Answer from the drawing. Dimensions are ordinates in mm from the lowest x, y and z of the part. A direction names the side the tool comes from. Coordinates: 2 decimals unless noted, no trailing zeros. Order: outer loops, then holes, each group sorted by start corner. A loop starts at its lowest first (then second) coordinate and runs counter-clockwise, first axis right, second up. Notation, with made-up numbers: (-13.5, 70.5) -> (31.5, 70.5) arc R22 cw to (31.5, 100.5) -> close; hole circle Ø11 at (-36, 82). An arc over 180 degrees is marked (long way). Answer in a Markdown table with one row per item.
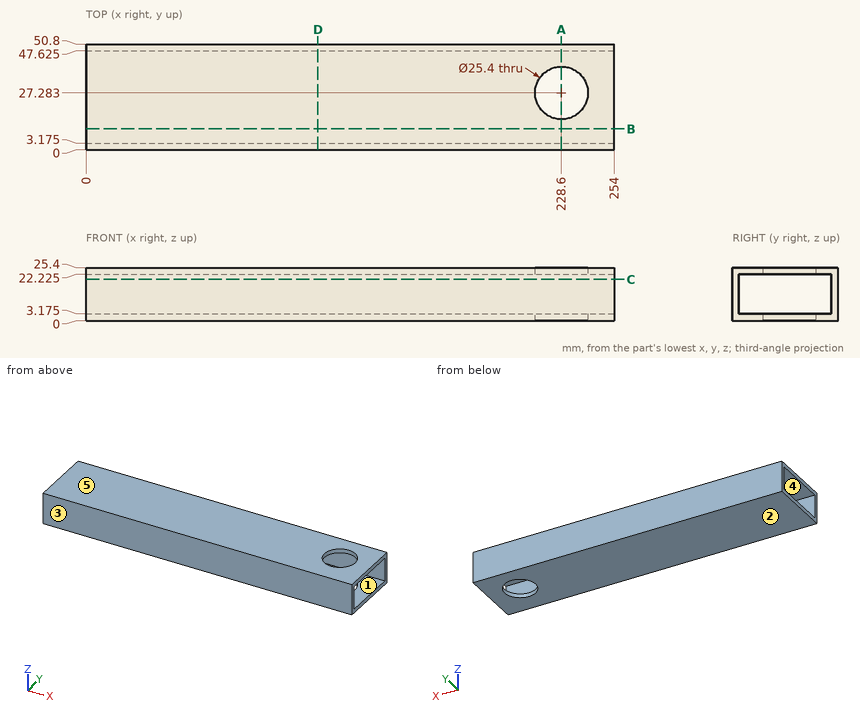
Q1. The part is cut by section C-C (z = 19.75). Write down the section's boundary in (x, y) (1 decimal), then the cut area to 3 significant figures.
Outcome:
| item | result |
|---|---|
| outline | (0, 0) -> (254, 0) -> (254, 3.2) -> (0, 3.2) -> close; (0, 47.6) -> (254, 47.6) -> (254, 50.8) -> (0, 50.8) -> close |
| area | 1,610 mm² |
Q2. The part is cut by section B-B (y = 10). Write down the section's boundary in (x, z) (1 decimal).
Outcome:
| item | result |
|---|---|
| outline | (0, 0) -> (254, 0) -> (254, 3.2) -> (0, 3.2) -> close; (0, 22.2) -> (254, 22.2) -> (254, 25.4) -> (0, 25.4) -> close |
Q3. Consider line 1 (Y direction, x = 140.5, z = 4) (1 decimal); line 2 (Y direction, x = 228.6, z = 23.5); line 3 (Z direction, x = 168, y = 30) (1 decimal). Determine where each line is inside the solid, lowest interval first.
Outcome:
| item | result |
|---|---|
| line 1 | 0 to 3.2, 47.6 to 50.8 |
| line 2 | 0 to 14.58, 39.98 to 50.8 |
| line 3 | 0 to 3.2, 22.2 to 25.4 |
Q4. The part is cut by section A-A (x = 228.6). Write down the section's boundary in (y, z) (1 decimal), then the cut area to 3 significant figures.
Outcome:
| item | result |
|---|---|
| outline | (0, 0) -> (14.6, 0) -> (14.6, 3.2) -> (3.2, 3.2) -> (3.2, 22.2) -> (14.6, 22.2) -> (14.6, 25.4) -> (0, 25.4) -> close; (40, 0) -> (50.8, 0) -> (50.8, 25.4) -> (40, 25.4) -> (40, 22.2) -> (47.6, 22.2) -> (47.6, 3.2) -> (40, 3.2) -> close |
| area | 282 mm² |
Q5. For the marked faces 1 and 2, determine the directions among +Z, -Z, +X, -X, +Y, -Y from which every point of the face is accessible in a straight line to the end or side of a thin tool.
Outcome:
| item | result |
|---|---|
| face 1 | +X, -X |
| face 2 | -Z, +X, -X, +Y, -Y |
Q6. For a pull along Z with two mould halves and no side action, classify the marked faces 3, 4 and 5 as pulls with the +Z half, pulls with the -Z half, needs draft (parallel to the pull), parting line crosses it, or undercut.
Outcome:
| item | result |
|---|---|
| face 3 | needs draft |
| face 4 | undercut |
| face 5 | pulls with the +Z half |
Q7. The part is cut by section D-D (x = 111.5). Write down the section's boundary in (y, z) (1 decimal).
Outcome:
| item | result |
|---|---|
| outline | (0, 0) -> (50.8, 0) -> (50.8, 25.4) -> (0, 25.4) -> close; hole (3.2, 3.2) -> (47.6, 3.2) -> (47.6, 22.2) -> (3.2, 22.2) -> close |
